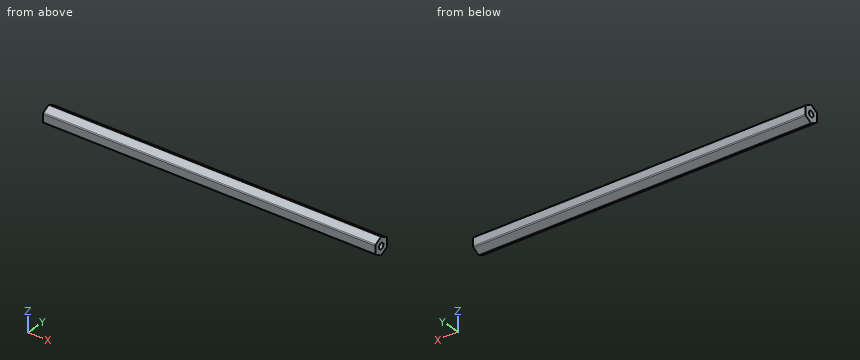
from build123d import *

# Parameters (mm, degrees)
SKETCH1_R           = 2.38125
BOSS_EXTRUDE1_DEPTH = 279.4


with BuildPart() as part:
    # Sketch1 → Boss-Extrude1 (new body)
    with BuildSketch(Plane(origin=(0, 0, 0), x_dir=(0, 0, -1), z_dir=(1, 0, 0))):
        with BuildLine():
            Line((7.039054482, 0.508), (3.959468146, 5.842))
            ThreePointArc((3.959468146, 5.842), (3.587586336, 6.21388181), (3.079586336, 6.35))
            Line((3.079586336, 6.35), (-3.079586336, 6.35))
            ThreePointArc((-3.079586336, 6.35), (-3.587586336, 6.21388181), (-3.959468146, 5.842))
            Line((-3.959468146, 5.842), (-7.039054482, 0.508))
            ThreePointArc((-7.039054482, 0.508), (-7.175172672, 0), (-7.039054482, -0.508))
            Line((-7.039054482, -0.508), (-3.959468146, -5.842))
            ThreePointArc((-3.959468146, -5.842), (-3.587586336, -6.21388181), (-3.079586336, -6.35))
            Line((-3.079586336, -6.35), (3.079586336, -6.35))
            ThreePointArc((3.079586336, -6.35), (3.587586336, -6.21388181), (3.959468146, -5.842))
            Line((3.959468146, -5.842), (7.039054482, -0.508))
            ThreePointArc((7.039054482, -0.508), (7.175172672, 0), (7.039054482, 0.508))
        make_face()
        Circle(SKETCH1_R, mode=Mode.SUBTRACT)
    extrude(amount=BOSS_EXTRUDE1_DEPTH)


solid = part.part
Read the model definition and answer for the solid it produces. Units are mm, in the model's axes. Coordinates: 2 decimals unless noted, no trailing zeros. Loops run counter-clockwise (first coordinate to the right, second up) from the corner with the lowest first, then second, coordinate; pieces in that order, holes last.
Q1. The part is cut by section A-A on x = 29. Write down the section's boundary in (y, z).
Q2. Consider probe 1 along Y at (x, z) = (175.5, 0); probe 2 along Z at (x, y) = (78, -0.25); probe 3 along Z at (x, y) = (181, 5.75). Determine where each line is inside the solid, lowest interval first.
Q3. The part is cut by section B-B on z = 0. Write down the section's boundary in (x, y), and give its area (3 significant figures).
Q4. Each of these flat-tipped pins is pushed along its axis until it touches: pin 1 Ø1 at (x, y) = (190.5, -3.5) entering from -Z; pin 2 Ø4.5 at (y, z) = (0, 0) entering from +X. Where does it stop, or does it pass through?
Results below:
1. outline: (-6.35, -3.08) arc R1.02 ccw to (-5.84, -3.96) - (-0.51, -7.04) arc R1.02 ccw to (0.51, -7.04) - (5.84, -3.96) arc R1.02 ccw to (6.35, -3.08) - (6.35, 3.08) arc R1.02 ccw to (5.84, 3.96) - (0.51, 7.04) arc R1.02 ccw to (-0.51, 7.04) - (-5.84, 3.96) arc R1.02 ccw to (-6.35, 3.08) - close; hole circle Ø4.76 at (0, 0)
2. probe 1: y = -6.35 to -2.38, 2.38 to 6.35
2. probe 2: z = -7.14 to -2.37, 2.37 to 7.14
2. probe 3: z = -4.01 to 4.01
3. outline: (0, -6.35) - (279.4, -6.35) - (279.4, -2.38) - (0, -2.38) - close; (0, 2.38) - (279.4, 2.38) - (279.4, 6.35) - (0, 6.35) - close
3. area: 2,220 mm2
4. pin 1: stops at z = -5.6
4. pin 2: passes through
